from build123d import *

# Parameters (mm, degrees)
BOSS_EXTRUDE1_DEPTH = 60
TAP2_D              = 3.242
TAP2_DEPTH          = 10.1
TAP2_TIP            = 0.973995063


with BuildPart() as part:
    # Sketch1 → Boss-Extrude1 (new body)
    with BuildSketch(Plane(origin=(0, 0, 0), x_dir=(0, 0, -1), z_dir=(1, 0, 0))):
        Polygon((0, 4.041451884), (-3.5, 2.020725942), (-3.5, -2.020725942), (0, -4.041451884), (3.5, -2.020725942), (3.5, 2.020725942), align=None)
    extrude(amount=BOSS_EXTRUDE1_DEPTH)

    # Sketch2 → Cut-Revolve1 (revolve, cut)
    with BuildSketch(Plane.XY):
        Polygon((0, 4.041451884), (0, 3.5), (0.312607391, 4.041451884), align=None)
        Polygon((59.687392609, 4.041451884), (60, 4.041451884), (60, 3.5), align=None)
    revolve(axis=Axis((0, 0, 0), (1, 0, 0)), mode=Mode.SUBTRACT)

    # Sketch6 → Revolve2 (revolve)
    with BuildSketch(Plane.XY):
        Polygon((0, 0), (0, 1.6), (-1.2, 1.6), (-1.2, 2), (-6, 2), (-6, 0), align=None)
    revolve(axis=Axis((0, 0, 0), (-1, 0, 0)))

    # Tap2
    with Locations(Plane(origin=(60, 0, 0), x_dir=(0, 0, -1), z_dir=(1, 0, 0))):
        with Locations((0, 0)):
            Hole(TAP2_D / 2, depth=TAP2_DEPTH)
            with Locations((0, 0, -(TAP2_DEPTH + TAP2_TIP / 2))):  # 118° drill point
                Cone(0, TAP2_D / 2, TAP2_TIP, mode=Mode.SUBTRACT)


solid = part.part
The listing builds one solid part. Answer for the finished solid, in the listing's coordinates (mm). A direction names the side the tool comes from. Round coordinates to 2 decimals unless told otherwise and drop trailing zeros. Order: outer loops, then holes, each group sorted by start corner. A loop starts at its lowest first (then second) coordinate and runs counter-clockwise, first axis right, second up. Notation, with made-up numbers: (23, 14) -> (41, 14) arc R20 ccw to (41, 42) -> close; hole circle Ø10 at (81.5, 26.5). An arc over 180 degrees is marked (long way). Put each result on its own line as item: value.
Q1. Consider line 1 along Z through (x, y) = (54.5, 0); line 2 along X through (y, z) = (2, -1.5); line 3 along Y through (x, z) = (0.5, 1.75). Determine where each line is inside the solid, lowest interval first.
Results list:
line 1: -3.5 to -1.62, 1.62 to 3.5
line 2: 0 to 60
line 3: -3.03 to 3.03
Q2. Each of these flat-tipped pins is pushed along its axis until it touches: P1, Ø2, axis at y = 0.5, z = 0, coming from the +X side; P2, Ø1.5, axis at x = 27.5, z = 2, coming from the +Y side. Where does it stop, or does it pass through?
Results list:
P1: x = 49.83
P2: y = 3.32
Q3. Section A-A, the plane x = 3.5 is taken. Write down the section's boundary in (y, z), and give its area (3 significant figures).
Results list:
outline: (-4.04, 0) -> (-2.02, -3.5) -> (2.02, -3.5) -> (4.04, 0) -> (2.02, 3.5) -> (-2.02, 3.5) -> close
area: 42.4 mm^2
Q4. Determine the mould class of faces 1 (the cylindrical face through (-0.61, -1.27, 0.97)), 2 (the conical face through (59.924, 1.808, -3.149)), 3 (the conical face through (49.095, -0.275, 0.061)) for opening direction Z: pulls with the +Z half, pulls with the -Z half, needs draft (parallel to the pull), parting line crosses it, or undercut.
Results list:
face 1: parting line crosses it
face 2: pulls with the -Z half
face 3: undercut
Q5. Which of the six approach directions +Z, -Z, +X, -X, +Y, -Y give full straight-line access (tool end or side, diameter ignored) to faces 4 (the cylindrical face through (54.879, -1.438, 0.748)), 5 (the conical face through (0.076, 3.632, -0.009)), 6 (the flat face through (0, -2, -1))?
Results list:
face 4: +X
face 5: -X, +Y
face 6: none
